Work out the finished part from the listing and answer in its coordinate system (mm). Face numbers are marked on the shaded views. A direction names the side the tool comes from. Coordinates: 2 decimals unless noted, no trailing zeros. Loops run counter-clockwise (first coordinate to the right, second up) from the corner with the lowest first, then second, coordinate; pieces in that order, holes last. Notation, with made-up numbers: M 78,43.5 L 105,43.5 A25 cw 105,56.5 Z; hole C 40,44.5 d11. An arc over 180 degrees is marked long. Write each question's results on one line, items separated by ' | '.
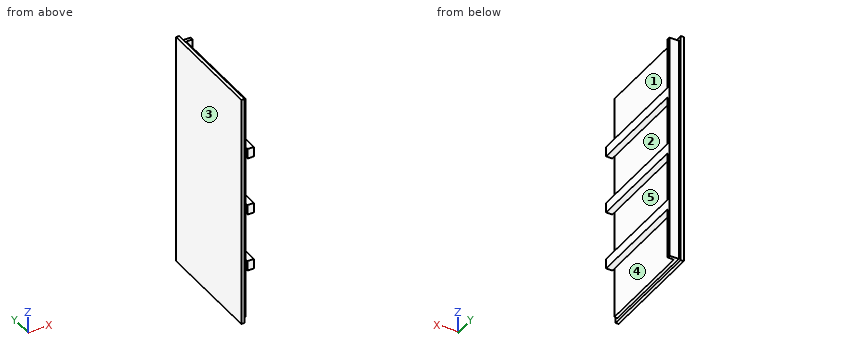
Autodesk Inventor part; units mm, degrees
ref_plane "YZ Plane" through (0, 0, 0) normal (1, 0, 0) x (0, 1, 0)
ref_plane "XZ Plane" through (0, 0, 0) normal (0, 1, 0) x (-1, 0, 0)
ref_plane "XY Plane" through (0, 0, 0) normal (0, 0, 1) x (1, 0, 0)
sketch "Sketch1" plane through (0, 0, 0) normal (1, 0, 0) x (0, 1, 0)
  line L0 (0, 0) -> (69.85, 0)
  line L1 (69.85, 0) -> (69.85, -150.4)
  line L2 (69.85, -150.4) -> (0, -150.4)
  line L3 (0, -150.4) -> (0, 0)
  dimension "d0" = 69.85
  dimension "d1" = 150.4
extrude "Extrusion1" add sketch "Sketch1" along normal blind 2
sketch "Sketch2" plane through (2, 0, 0) normal (1, 0, 0) x (0, 0, -1)
  line L0 (150.4, 0) -> (150.4, 69.85)
  line L1 (150.4, 69.85) -> (0, 69.85)
  line L2 (0, 69.85) -> (0, 0)
  line L3 (0, 0) -> (150.4, 0)
  line L4 (150.4, 69.85) -> (148.4, 69.85)
  line L5 (148.4, 69.85) -> (148.4, 0)
  line L6 (148.4, 0) -> (150.4, 0)
  line L7 (150.4, 0) -> (150.4, 69.85)
  line L8 (0, 69.85) -> (2, 69.85)
  line L9 (2, 69.85) -> (2, 0)
  line L10 (2, 0) -> (0, 0)
  line L11 (0, 0) -> (0, 69.85)
  line L12 (0, 0) -> (150.4, 0)
  line L13 (150.4, 0) -> (150.4, 2)
  line L14 (150.4, 2) -> (0, 2)
  line L15 (0, 2) -> (0, 0)
  point P0 (2, 2)
  point P1 (148.4, 2)
  dimension "d4" = 2
  dimension "d5" = 2
  dimension "d6" = 2
extrude "Extrusion2" add sketch "Sketch2" along normal blind 2 contours L14 L9 L1 L5
sketch "Sketch3" plane through (4, 0, 0) normal (1, 0, 0) x (0, 0, -1)
  line L0 (150.4, 0) -> (150.4, 69.85)
  line L1 (0, 0) -> (150.4, 0)
  line L2 (0, 69.85) -> (0, 0)
  line L3 (150.4, 69.85) -> (0, 69.85)
  line L4 (0, 69.85) -> (75.2, 69.85) construction
  line L5 (75.2, 69.85) -> (75.2, 0) construction
  line L6 (75.2, 0) -> (0, 0) construction
  line L7 (0, 0) -> (0, 69.85) construction
  line L8 (0, 0) -> (150.4, 0) construction
  line L9 (0, 0) -> (37.6, 0) construction
  line L10 (37.6, 0) -> (37.6, 69.85) construction
  line L11 (37.6, 69.85) -> (0, 69.85) construction
  line L12 (0, 69.85) -> (0, 0) construction
  line L13 (150.4, 0) -> (150.4, 69.85) construction
  line L14 (75.2, 69.85) -> (150.4, 69.85) construction
  line L15 (150.4, 69.85) -> (150.4, 0) construction
  line L16 (150.4, 0) -> (75.2, 0) construction
  line L17 (75.2, 0) -> (75.2, 69.85) construction
  line L18 (75.2, 0) -> (112.8, 0) construction
  line L19 (112.8, 0) -> (112.8, 69.85) construction
  line L20 (112.8, 69.85) -> (75.2, 69.85) construction
  line L21 (75.2, 69.85) -> (75.2, 0) construction
  line L22 (34.425, 0) -> (34.425, 69.85) construction
  line L23 (34.425, 69.85) -> (40.775, 69.85) construction
  line L24 (40.775, 69.85) -> (40.775, 0) construction
  line L25 (40.775, 0) -> (34.425, 0) construction
  line L26 (34.425, 0) -> (40.775, 69.85) construction
  line L27 (34.425, 69.85) -> (40.775, 0) construction
  line L28 (72.025, 0) -> (72.025, 69.85) construction
  line L29 (72.025, 69.85) -> (78.375, 69.85) construction
  line L30 (78.375, 69.85) -> (78.375, 0) construction
  line L31 (78.375, 0) -> (72.025, 0) construction
  line L32 (72.025, 0) -> (78.375, 69.85) construction
  line L33 (72.025, 69.85) -> (78.375, 0) construction
  line L34 (109.625, 0) -> (109.625, 69.85) construction
  line L35 (109.625, 69.85) -> (115.975, 69.85) construction
  line L36 (115.975, 69.85) -> (115.975, 0) construction
  line L37 (115.975, 0) -> (109.625, 0) construction
  line L38 (109.625, 0) -> (115.975, 69.85) construction
  line L39 (109.625, 69.85) -> (115.975, 0) construction
  line L40 (34.425, 69.85) -> (40.775, 69.85)
  line L41 (40.775, 69.85) -> (40.775, 0)
  line L42 (40.775, 0) -> (34.425, 0)
  line L43 (34.425, 0) -> (34.425, 69.85)
  line L44 (72.025, 0) -> (78.375, 0)
  line L45 (78.375, 0) -> (78.375, 69.85)
  line L46 (78.375, 69.85) -> (72.025, 69.85)
  line L47 (72.025, 69.85) -> (72.025, 0)
  line L48 (109.625, 69.85) -> (115.975, 69.85)
  line L49 (115.975, 69.85) -> (115.975, 0)
  line L50 (115.975, 0) -> (109.625, 0)
  line L51 (109.625, 0) -> (109.625, 69.85)
  point P0 (37.6, 34.925)
  point P1 (75.2, 34.925)
  point P2 (112.8, 34.925)
  dimension "d9" = 6.35
  dimension "d10" = 6.35
  dimension "d11" = 6.35
extrude "Extrusion3" add sketch "Sketch3" along normal blind 4 contours L1 L51 L3 L49 | L1 L47 L3 L45 | L1 L43 L3 L41
sketch "Sketch4" plane through (0, 69.85, 0) normal (0, 1, 0) x (1, 0, 0)
  line L0 (0, 150.4) -> (0, 0)
  line L1 (0, 150.4) -> (0, 0) construction
  line L2 (0, 0) -> (2, 0) construction
  line L3 (2, 2) -> (2, 0) construction
  line L4 (2, 2) -> (4, 2) construction
  line L5 (4, 34.425) -> (4, 2) construction
  line L6 (4, 34.425) -> (8, 34.425) construction
  line L7 (8, 40.775) -> (8, 34.425) construction
  line L8 (4, 40.775) -> (8, 40.775) construction
  line L9 (4, 72.025) -> (4, 40.775) construction
  line L10 (4, 72.025) -> (8, 72.025) construction
  line L11 (8, 78.375) -> (8, 72.025) construction
  line L12 (4, 78.375) -> (8, 78.375) construction
  line L13 (4, 109.625) -> (4, 78.375) construction
  line L14 (4, 109.625) -> (8, 109.625) construction
  line L15 (8, 115.975) -> (8, 109.625) construction
  line L16 (4, 115.975) -> (8, 115.975) construction
  line L17 (4, 148.4) -> (4, 115.975) construction
  line L18 (2, 148.4) -> (4, 148.4) construction
  line L19 (2, 150.4) -> (2, 148.4) construction
  line L20 (0, 150.4) -> (2, 150.4) construction
  line L21 (2, 0) -> (0, 0)
  line L22 (0, 0) -> (0, 150.4)
  line L23 (0, 150.4) -> (2, 150.4)
  line L24 (2, 150.4) -> (2, 0)
  line L25 (2, 0) -> (8, 0)
  line L26 (8, 0) -> (8, 150.4)
  line L27 (8, 150.4) -> (2, 150.4)
  line L28 (2, 150.4) -> (2, 0)
extrude "Extrusion4" cut sketch "Sketch4" against normal blind 2 contours L27 L26 L25 L24
sketch "Sketch5" plane through (0, 67.85, 0) normal (0, 1, 0) x (1, 0, 0)
  line L0 (4, 115.975) -> (8, 115.975)
  line L1 (4, 148.4) -> (4, 115.975)
  line L2 (2, 148.4) -> (4, 148.4)
  line L3 (2, 2) -> (2, 148.4)
  line L4 (4, 2) -> (2, 2)
  line L5 (4, 34.425) -> (4, 2)
  line L6 (8, 34.425) -> (4, 34.425)
  line L7 (8, 40.775) -> (8, 34.425)
  line L8 (4, 40.775) -> (8, 40.775)
  line L9 (4, 72.025) -> (4, 40.775)
  line L10 (8, 72.025) -> (4, 72.025)
  line L11 (8, 78.375) -> (8, 72.025)
  line L12 (4, 78.375) -> (8, 78.375)
  line L13 (4, 109.625) -> (4, 78.375)
  line L14 (8, 109.625) -> (4, 109.625)
  line L15 (8, 115.975) -> (8, 109.625)
  line L16 (2, 2) -> (4, 2)
  line L17 (2, 2) -> (8, 2)
  line L18 (8, 2) -> (8, 148.4)
  line L19 (8, 148.4) -> (2, 148.4)
  line L20 (2, 148.4) -> (2, 2)
  point P0 (0, 0)
  point P1 (4, 2)
extrude "Extrusion5" add sketch "Sketch5" against normal blind 2 contours L1 L19 L18 L0 | L18 L12 L13 L14 | L18 L8 L9 L10 | L5 L6 L18 L17
properties part number "leftwall"
1) Which of the six approach directions +Z, -Z, +X, -X, +Y, -Y give full straight-line access (tool end or side, diameter ignored) to the marked faces 3, 4 and 5?
Check result:
face 3: +Z, -Z, -X, +Y, -Y | face 4: -Z, +X, -Y | face 5: +X, -Y
2) Straight lines are drawn through the part: probe 1 along Z at (x, y) = (6.5, 32.5) (3 decimals); probe 2 along Y at (x, z) = (3.25, -142); probe 3 along Y at (x, z) = (6.75, -27.5). For each, find the intervals that lie inside material, in ascending order. Write a range as [from, to].
Check result:
probe 1: [-115.975, -109.625], [-78.375, -72.025], [-40.775, -34.425] | probe 2: [2, 67.85] | probe 3: [65.85, 67.85]
3) Find section C-C, the plane x = 5.25. Give the vertices of the cut face in (y, z) (3 decimals).
Check result:
outline: M 0,-115.975 L 65.85,-115.975 L 65.85,-148.4 L 67.85,-148.4 L 67.85,-2 L 65.85,-2 L 65.85,-34.425 L 0,-34.425 L 0,-40.775 L 65.85,-40.775 L 65.85,-72.025 L 0,-72.025 L 0,-78.375 L 65.85,-78.375 L 65.85,-109.625 L 0,-109.625 Z
4) Find section B-B, the plane y = 52.5. Give the vertices of the cut face in (x, z) (3 decimals), and give its area (3 significant figures).
Check result:
outline: M 0,-150.4 L 2,-150.4 L 2,-148.4 L 4,-148.4 L 4,-115.975 L 8,-115.975 L 8,-109.625 L 4,-109.625 L 4,-78.375 L 8,-78.375 L 8,-72.025 L 4,-72.025 L 4,-40.775 L 8,-40.775 L 8,-34.425 L 4,-34.425 L 4,-2 L 2,-2 L 2,0 L 0,0 Z | area: 670 mm^2
5) Find section A-A, the plane z = -133. Give the vertices of the cut face in (x, y), and give its area (3 significant figures).
Check result:
outline: M 0,0 L 2,0 L 2,2 L 4,2 L 4,65.85 L 8,65.85 L 8,67.85 L 2,67.85 L 2,69.85 L 0,69.85 Z | area: 279 mm^2
6) For a pull along Z with two mould halves and no side action, classify the marked faces 1 and 2 as released by +Z, released by -Z, zero draft, split by the parting line, or undercut.
Check result:
face 1: zero draft | face 2: undercut
7) Given pin 1 Ø1.2 at (x, y) = (6, 44.5) entering from -Z (3 decimals); pin 2 Ø3 at (x, y) = (5, 36.5) entering from +Z; pin 3 Ø1.8 at (x, z) = (4, -52.5) entering from +Y, each flat-ended and moving along its own axis, determine where each tip first touches the part or whether it passes through.
Check result:
pin 1: z = -115.975 | pin 2: z = -2 | pin 3: y = 67.85
